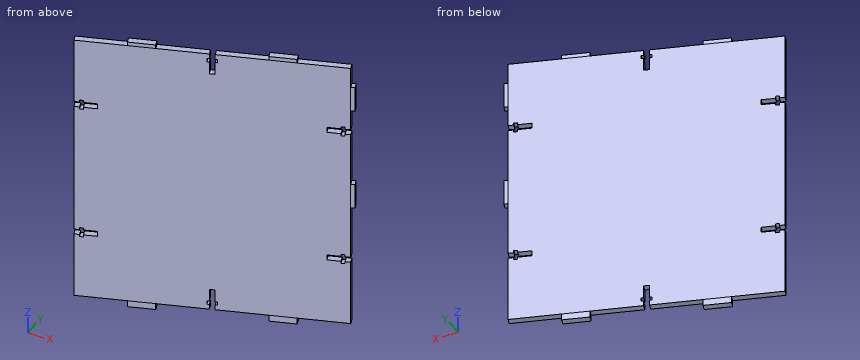
from build123d import *

# Parameters (mm, degrees)
BOSS_EXTRUDE1_DEPTH = 217.2
CUT_EXTRUDE3_DEPTH  = 68.63050203
SKETCH5_W           = 20
SKETCH5_H           = 5
SKETCH5_W_2         = 3
SKETCH5_H_2         = 20
SKETCH5_H_3         = 3
BOSS_EXTRUDE2_DEPTH = 5


with BuildPart() as part:
    # Sketch2 → Boss-Extrude1 (new body)
    with BuildSketch(Plane.XY.offset(2)):
        Polygon((29.309289207, -6.943664177), (31.018091452, -11.642599682), (-152.24039327, -78.285887246), (-153.949195515, -73.586951741), align=None)
    extrude(amount=BOSS_EXTRUDE1_DEPTH)

    # Sketch4 → Cut-Extrude3 (cut, through all)
    with BuildSketch(Plane(origin=(7.362313595, -20.245196221, 0), x_dir=(-0.939787101, -0.341760449, 0), z_dir=(0.341760449, -0.939787101, 0))):
        Polygon((70.228577846, -2), (74.428577846, -2), (74.428577846, -6), (76.128577846, -6), (76.128577846, -8.8), (74.428577846, -8.8), (74.428577846, -18.8), (70.228577846, -18.8), (70.228577846, -8.8), (68.528577846, -8.8), (68.528577846, -6), (70.228577846, -6), align=None)
        Polygon((-25.171422154, -58.4), (-25.171422154, -54.2), (-21.171422154, -54.2), (-21.171422154, -52.5), (-18.371422154, -52.5), (-18.371422154, -54.2), (-8.371422154, -54.2), (-8.371422154, -58.4), (-18.371422154, -58.4), (-18.371422154, -60.1), (-21.171422154, -60.1), (-21.171422154, -58.4), align=None)
        Polygon((74.428577846, -219.2), (70.228577846, -219.2), (70.228577846, -215.2), (68.528577846, -215.2), (68.528577846, -212.4), (70.228577846, -212.4), (70.228577846, -202.4), (74.428577846, -202.4), (74.428577846, -212.4), (76.128577846, -212.4), (76.128577846, -215.2), (74.428577846, -215.2), align=None)
        Polygon((-21.171422154, -167), (-21.171422154, -168.7), (-18.371422154, -168.7), (-18.371422154, -167), (-8.371422154, -167), (-8.371422154, -162.8), (-18.371422154, -162.8), (-18.371422154, -161.1), (-21.171422154, -161.1), (-21.171422154, -162.8), (-25.171422154, -162.8), (-25.171422154, -167), align=None)
        Polygon((169.828577846, -162.8), (169.828577846, -167), (165.828577846, -167), (165.828577846, -168.7), (163.028577846, -168.7), (163.028577846, -167), (153.028577846, -167), (153.028577846, -162.8), (163.028577846, -162.8), (163.028577846, -161.1), (165.828577846, -161.1), (165.828577846, -162.8), align=None)
        Polygon((165.828577846, -54.2), (165.828577846, -52.5), (163.028577846, -52.5), (163.028577846, -54.2), (153.028577846, -54.2), (153.028577846, -58.4), (163.028577846, -58.4), (163.028577846, -60.1), (165.828577846, -60.1), (165.828577846, -58.4), (169.828577846, -58.4), (169.828577846, -54.2), align=None)
    extrude(amount=-CUT_EXTRUDE3_DEPTH, mode=Mode.SUBTRACT)

    # Sketch5 → Boss-Extrude2 (add)
    with BuildSketch(Plane(origin=(7.362313595, -20.245196221, 0), x_dir=(0.939787101, 0.341760449, 0), z_dir=(0.341760449, -0.939787101, 0))):
        with Locations((-22.528577846, -0.5)):
            Rectangle(SKETCH5_W, SKETCH5_H)
        with Locations((-122.128577846, -0.5)):
            Rectangle(SKETCH5_W, SKETCH5_H)
        with Locations((26.671422154, 110.6)):
            Rectangle(SKETCH5_W_2, SKETCH5_H_2)
        with Locations((26.671422154, 193.1)):
            Rectangle(SKETCH5_W_2, SKETCH5_H_2)
        with Locations((-22.528577846, 220.7)):
            Rectangle(SKETCH5_W, SKETCH5_H_3)
        with Locations((-122.128577846, 220.7)):
            Rectangle(SKETCH5_W, SKETCH5_H_3)
    extrude(amount=-BOSS_EXTRUDE2_DEPTH)


solid = part.part
Could you check a few things on this model? Use its own coordinates, in mm. Give positions to 0.01 mm unless a question says otherwise; leave off trailing zeros. Order: outer loops, then holes, each group sorted by start corner. A loop starts at its lowest first (then second) coordinate and runs counter-clockwise, first axis right, second up. Notation, with made-up numbers: (24, 7) - (52, 7) arc R18 ccw to (52, 30) - close; hole circle Ø8 at (38, 1). An arc over 180 degrees is marked (long way). Return JSON: item names as keys, results as strings. Group by question number.
Q1. Suppose I cut it at D-D, the plane y = -50.5. Please give me the cut outline in (x, z), and give its area (3 significant figures).
Q2. Will these pins go through, and if not, where does the flat tip stop? pin 1 Ø2.5 at (x, y) = (27, -10) entering from -Z; pin 2 Ø1 at (x, y) = (-64.5, -44.5) entering from +Z; pin 3 Ø4 at (x, z) = (-44, 30) entering from +Y.
Q3. Suppose I cut it at A-A, the plane z = 16. Please give me the cut outline in (x, y), and give its area (3 significant figures).
Q4. Suppose I cut it at C-C, the plane z = 113. Please give me the cut outline in (x, y).
Q5. Please list where these lines run through material, in increasing order: line 1 along Y through (x, z) = (5, 153); line 2 along Y through (x, z) = (-93.5, 212.5). Write a range as [from, to].
Q6. Suppose I cut it at B-B, the plane x = 20. Please give me the cut outline in (y, z), and give its area (3 significant figures).
Resolved:
{
 "1": {"outline": "(-90.46, 2) - (-75.83, 2) - (-75.83, 219.2) - (-90.46, 219.2) - close", "area": "3,180 mm2"},
 "2": {"pin 1": "stops at z = 2", "pin 2": "stops at z = 219.2", "pin 3": "stops at y = -32.88"},
 "3": {"outline": "(-153.95, -73.59) - (-152.24, -78.29) - (-62.58, -45.68) - (-64.29, -40.98) - close; (-60.35, -39.55) - (-58.64, -44.25) - (31.02, -11.64) - (29.31, -6.94) - close", "area": "954 mm2"},
 "4": {"outline": "(-153.95, -73.59) - (-152.24, -78.29) - (33.84, -10.62) - (32.13, -5.92) - close"},
 "5": {"line 1": "y = [-21.1, -15.78]", "line 2": "y = [-56.92, -51.6]"},
 "6": {"outline": "(-15.65, 2) - (-10.33, 2) - (-10.33, 54.2) - (-15.65, 54.2) - close; (-15.65, 58.4) - (-10.33, 58.4) - (-10.33, 162.8) - (-15.65, 162.8) - close; (-15.65, 167) - (-10.33, 167) - (-10.33, 219.2) - (-15.65, 219.2) - close", "area": "1,110 mm2"}
}
